```python
from build123d import *

# Parameters (mm, degrees)
F0_R     = 1.5875
F1_DEPTH = 3.048


# Not quite as in the source:
# - ends of sketch curves that miss each other by under 0.0002 mm in the source are joined


with BuildPart() as f1:
    # F0 (on Front) → F1 (new body)
    with BuildSketch(Plane.XZ):
        with BuildLine():
            ThreePointArc((-20.4063861121, 50.6759697353), (-20.4057804387, 50.7379835531), (-20.4055785447, 50.8))
            ThreePointArc((-20.4055785447, 50.8), (-29.9930844021, 60.3247949069), (-39.454758181, 50.6749909771))
            ThreePointArc((-39.454758181, 50.6749909771), (-36.6214272972, 44.0207546164), (-29.9305785447, 41.275))
            ThreePointArc((-29.9305785447, 41.275), (-23.2393814647, 44.0210984197), (-20.4063861121, 50.6759697353))
        make_face()
        with BuildLine():
            ThreePointArc((-26.7555785447, 50.8), (-27.6855145145, 48.5549359697), (-29.9305785447, 47.625))
            ThreePointArc((-29.9305785447, 47.625), (-32.175642575, 53.0450640303), (-26.7555785447, 50.8))
        make_face(mode=Mode.SUBTRACT)
        with BuildLine():
            ThreePointArc((-29.9305785447, 41.275), (-36.6214272972, 44.0207546164), (-39.454758181, 50.6749909771))
            Line((-39.454758181, 50.6749909771), (-45.6773538826, 2.0136264451))
            ThreePointArc((-45.6773538826, 2.0136264451), (-40.4198422268, 11.9159964924), (-29.9305785447, 15.875))
            Line((-29.9305785447, 15.875), (-29.9305785447, 41.275))
        make_face()
        with Locations((-33.3938002586, 36.5252)):
            Circle(F0_R, mode=Mode.SUBTRACT)
        with BuildLine():
            Line((-14.1837976059, 2.0135826444), (-20.4063861121, 50.6759697353))
            ThreePointArc((-20.4063861121, 50.6759697353), (-23.2393814647, 44.0210984197), (-29.9305785447, 41.275))
            Line((-29.9305785447, 41.275), (-29.9305785447, 15.875))
            ThreePointArc((-29.9305785447, 15.875), (-19.4412982901, 11.9159819041), (-14.1837976059, 2.0135826444))
        make_face()
        with BuildLine():
            ThreePointArc((-29.9305785447, 15.875), (-40.4198422268, 11.9159964924), (-45.6773538826, 2.0136264451))
            ThreePointArc((-45.6773538826, 2.0136264451), (-45.8043998708, -0.1934463924), (-45.6236065946, -2.3967677453))
            ThreePointArc((-45.6236065946, -2.3967677453), (-40.2738598675, -12.0429297298), (-29.9305785447, -15.875))
            Line((-29.9305785447, -15.875), (-29.9305785447, -3.175))
            ThreePointArc((-29.9305785447, -3.175), (-33.1055785447, 0), (-29.9305785447, 3.175))
            Line((-29.9305785447, 3.175), (-29.9305785447, 15.875))
        make_face()
        with BuildLine():
            ThreePointArc((-14.0555785447, 0), (-14.087665738, 1.0088304111), (-14.1837976059, 2.0135826444))
            ThreePointArc((-14.1837976059, 2.0135826444), (-19.4412982901, 11.9159819041), (-29.9305785447, 15.875))
            Line((-29.9305785447, 15.875), (-29.9305785447, 3.175))
            ThreePointArc((-29.9305785447, 3.175), (-27.6855145145, 2.2450640303), (-26.7555785447, 0))
            ThreePointArc((-26.7555785447, 0), (-27.6855145145, -2.2450640303), (-29.9305785447, -3.175))
            Line((-29.9305785447, -3.175), (-29.9305785447, -15.875))
            ThreePointArc((-29.9305785447, -15.875), (-20.2346648726, -12.5699993263), (-14.5759167084, -4.031127))
            ThreePointArc((-14.5759167084, -4.031127), (-14.1862004743, -2.0322854558), (-14.0555785447, 0))
        make_face()
        with BuildLine():
            ThreePointArc((-29.9305785447, -15.875), (-40.2738598675, -12.0429297298), (-45.6236065946, -2.3967677453))
            Line((-45.6236065946, -2.3967677453), (-39.3767361242, -62.2769987798))
            ThreePointArc((-39.3767361242, -62.2769987798), (-36.2185248858, -56.3454660661), (-29.9305785447, -53.975))
            Line((-29.9305785447, -53.975), (-29.9305785447, -15.875))
        make_face()
        with BuildLine():
            ThreePointArc((-14.5759167084, -4.031127), (-20.2346648726, -12.5699993263), (-29.9305785447, -15.875))
            Line((-29.9305785447, -15.875), (-29.9305785447, -53.975))
            ThreePointArc((-29.9305785447, -53.975), (-23.1953864539, -56.7648079092), (-20.4055785447, -63.5))
            Line((-20.4055785447, -63.5), (6.5819214553, -63.5))
            ThreePointArc((6.5819214553, -63.5), (9.0069371863, -57.7889209921), (14.8002328719, -55.5674688026))
            Line((14.8002328719, -55.5674688026), (-11.021864061, -54.648172114))
            ThreePointArc((-11.021864061, -54.648172114), (-16.7206173005, -51.9399910767), (-18.6518593628, -45.9333000481))
            Line((-18.6518593628, -45.9333000481), (-14.5759167084, -4.031127))
        make_face()
        with BuildLine():
            ThreePointArc((-29.9305785447, -53.975), (-36.2185248858, -56.3454660661), (-39.3767361242, -62.2769987798))
            ThreePointArc((-39.3767361242, -62.2769987798), (-37.1496877578, -69.7137015675), (-30.1273622995, -73.0229670352))
            Line((-30.1273622995, -73.0229670352), (-29.0609056002, -72.9852144925))
            ThreePointArc((-29.0609056002, -72.9852144925), (-22.8946258802, -69.920357864), (-20.4055785447, -63.5))
            Line((-20.4055785447, -63.5), (-26.7555785447, -63.5))
            ThreePointArc((-26.7555785447, -63.5), (-32.175642575, -65.7450640303), (-29.9305785447, -60.325))
            Line((-29.9305785447, -60.325), (-29.9305785447, -53.975))
        make_face()
        with BuildLine():
            Line((-29.0609056002, -72.9852144925), (-30.1273622995, -73.0229670352))
            ThreePointArc((-30.1273622995, -73.0229670352), (-29.593604838, -73.0190374367), (-29.0609056002, -72.9852144925))
        make_face()
        with BuildLine():
            Line((6.5819214553, -63.5), (-20.4055785447, -63.5))
            ThreePointArc((-20.4055785447, -63.5), (-22.8946258802, -69.920357864), (-29.0609056002, -72.9852144925))
            Line((-29.0609056002, -72.9852144925), (14.8002328776, -71.4325311972))
            ThreePointArc((14.8002328776, -71.4325311972), (9.0069371884, -69.2110790099), (6.5819214553, -63.5))
        make_face()
        with BuildLine():
            ThreePointArc((14.8002328719, -55.5674688026), (9.0069371863, -57.7889209921), (6.5819214553, -63.5))
            ThreePointArc((6.5819214553, -63.5), (9.0069371884, -69.2110790099), (14.8002328776, -71.4325311972))
            ThreePointArc((14.8002328776, -71.4325311972), (20.2305004652, -69.0124842669), (22.4569214553, -63.5))
            ThreePointArc((22.4569214553, -63.5), (20.2305004632, -57.9875157311), (14.8002328719, -55.5674688026))
        make_face()
        with BuildLine():
            ThreePointArc((17.6944214553, -63.5), (14.5194214553, -66.675), (11.3444214553, -63.5))
            ThreePointArc((11.3444214553, -63.5), (14.5194214553, -60.325), (17.6944214553, -63.5))
        make_face(mode=Mode.SUBTRACT)
    extrude(amount=F1_DEPTH)


solid = f1.part
```
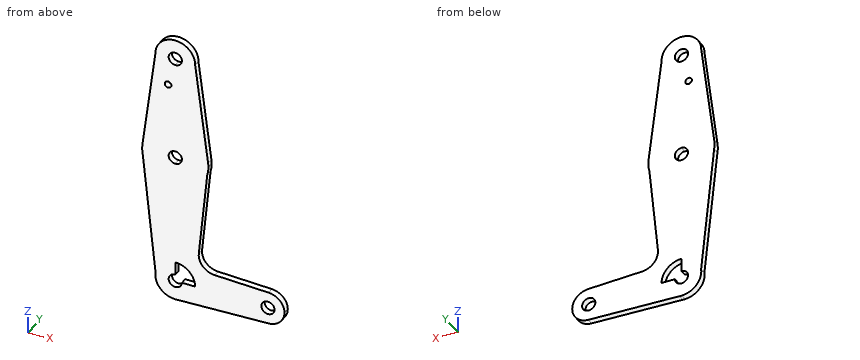
Part model, mm, in its own coordinate system. Give positions to 0.01 mm unless a question says otherwise; leave off trailing zeros. Write each loop counter-clockwise with the first axis right and the second up, starting at its lowest first coordinate (ties: lowest second). Pieces come first, ordered by that corner, then holes. Notation, with made-up numbers: (-11, 33) -> (47, 33) arc R17 cw to (47, 50) -> close; hole circle Ø5 at (45.5, 2). An arc over 180 degrees is marked (long way). Put each result on its own line as item: value. Start each with the question number.
Item 1: Cut at B-B (z = -49.5). List the corners of the cut face in (x, y), then the cut area to 3 significant figures.
Item 2: Pin check, flat tip, straight feed: pin 1 Ø0.9 at (x, y) = (-24.5, -2) entering from +Z. Stop position of the tip, or through.
Item 3: Wall check: L1, parallel to X at y = -0.65, z = 50.8; L2, parallel to Z at x = 14.5, y = -2.1; L3, parallel to Z at x = 15, y = -1.65. Give the ranges that are in metal, low to high. Write a range as [from, to].
Item 4: Cut at A-A (y = -2.35). State how many separate pieces and enclosed holes the cut face has, then the cut area to 3 significant figures.
Answer list:
1. outline: (-40.71, -3.05) -> (-18.18, -3.05) -> (-18.18, 0) -> (-40.71, 0) -> close
1. area: 68.7 mm2
2. pin 1: stops at z = 58.92
3. L1: x = [-39.46, -33.11], [-26.76, -20.41]
3. L2: z = [-71.44, -66.67], [-60.33, -55.56]
3. L3: z = [-71.42, -66.64], [-60.36, -55.58]
4. separate pieces: 1
4. enclosed holes: 5
4. area: 3,720 mm2
